Autodesk Inventor part; units mm, degrees
ref_plane "YZ Plane" through (0, 0, 0) normal (1, 0, 0) x (0, 1, 0)
ref_plane "XZ Plane" through (0, 0, 0) normal (0, 1, 0) x (-1, 0, 0)
ref_plane "XY Plane" through (0, 0, 0) normal (0, 0, 1) x (1, 0, 0)
sketch "Sketch1" plane through (0, 0, 0) normal (0, 0, 1) x (1, 0, 0)
  circle A0 centre (12.7, -88.9) radius 2.1844
  circle A1 centre (-149.225, -88.9) radius 2.1844
  circle A2 centre (12.7, -25.4) radius 2.1844
  circle A3 centre (-149.225, -25.4) radius 2.1844
  circle A4 centre (-149.225, -63.5) radius 2.1844
  circle A5 centre (12.7, -63.5) radius 2.1844
  line L0 (12.7, -19.05) -> (-149.225, -19.05)
  line L1 (-155.575, -25.4) -> (-155.575, -98.425)
  line L2 (-152.4, -101.6) -> (-140.7239, -101.6)
  line L3 (-138.1125, -100.2308) -> (-116.4997, -68.9766)
  line L4 (-106.054, -63.5) -> (-30.471, -63.5)
  line L5 (-20.0253, -68.9766) -> (1.5875, -100.2308)
  line L6 (4.1989, -101.6) -> (15.875, -101.6)
  line L7 (19.05, -98.425) -> (19.05, -25.4)
  arc A6 (19.05, -25.4) -> (12.7, -19.05) centre (12.7, -25.4) ccw
  arc A7 (-149.225, -19.05) -> (-155.575, -25.4) centre (-149.225, -25.4) ccw
  arc A8 (15.875, -101.6) -> (19.05, -98.425) centre (15.875, -98.425) ccw
  arc A9 (1.5875, -100.2308) -> (4.1989, -101.6) centre (4.1989, -98.425) ccw
  arc A10 (-140.7239, -101.6) -> (-138.1125, -100.2308) centre (-140.7239, -98.425) ccw
  arc A11 (-155.575, -98.425) -> (-152.4, -101.6) centre (-152.4, -98.425) ccw
  line L8 (-68.2625, -19.05) -> (-68.2625, -63.5) construction
  arc A12 (-20.0253, -68.9766) -> (-30.471, -63.5) centre (-30.471, -76.2) ccw
  arc A13 (-106.054, -63.5) -> (-116.4997, -68.9766) centre (-106.054, -76.2) ccw
  line L9 (-119.0625, -19.05) -> (-119.0625, 0)
  line L10 (-119.0625, 0) -> (-17.4625, 0)
  line L11 (-17.4625, 0) -> (-17.4625, -19.05)
  point P0 (0, 0)
  point P1 (-112.7125, -63.5)
  point P2 (-23.8125, -63.5)
  dimension "d0" = 6.35
  dimension "d2" = 3.175
  dimension "d3" = 12.7
  dimension "d4" = 88.9
  dimension "d5" = 44.45
  dimension "d6" = 25.4
  dimension "d7" = 12.7
  dimension "d23" = 101.6
  dimension "d24" = 19.05
extrude "Extrusion1" add sketch "Sketch1" along normal blind 6.35
fillet "Fillet2" radius 3.175 4 edges at (-119.0625, 0, 3.175) (-119.0625, -19.05, 3.175) (-17.4625, 0, 3.175) (-17.4625, -19.05, 3.175)
sketch "Sketch3" plane through (0, 0, 6.35) normal (0, 0, 1) x (1, 0, 0)
  circle A0 centre (12.7, -25.4) radius 2.1844
  circle A1 centre (12.7, -25.4) radius 4.7625
  circle A2 centre (12.7, -63.5) radius 2.1844
  circle A3 centre (12.7, -63.5) radius 4.7625
  circle A4 centre (-149.225, -25.4) radius 2.1844
  circle A5 centre (-149.225, -25.4) radius 4.7625
  circle A6 centre (-149.225, -63.5) radius 2.1844
  circle A7 centre (-149.225, -63.5) radius 4.7625
  point P0 (0, 0)
  dimension "d26" = 9.525
  dimension "d27" = 9.525
  dimension "d28" = 9.525
  dimension "d29" = 9.525
extrude "Extrusion3" cut sketch "Sketch3" against normal blind 3.175 contours A0 | A1 | A2 | A3 | A4 | A5 | A6 | A7
properties part number "backalignermidgoal" material "Acetal Resin, Black"
For this review, take the finished solid that the model builds, in its own axes (mm). A direction names the side the tool comes from. Round coordinates to 2 decimals unless told otherwise and drop trailing zeros. Write each loop counter-clockwise with the first axis right and the second up, starting at its lowest first coordinate (ties: lowest second). Pieces come first, ordered by that corner, then holes. Notation, with made-up numbers: M -6,33.5 L 19,33.5 A31 ccw 19,57.5 Z; hole C 25.5,2.5 d1. An arc over 180 degrees is marked long. One line per item, written item: value. Start each with the question number.
(1) We need section B-B (z = 4.5). Count the separate pieces of the cut face and the enclosed holes in it, and give its area (3 significant figures).
(2) We need section A-A (y = -79). Give the boundary of the cut face in (x, z) (3 decimals).
(3) The part is to be moulded in two halves that separate along X. For faces 1 (the cylindrical face through (-152.735, -60.281, 4.785)), 2 (the flat face through (-69, -39, 6.35)), 3 (the flat face through (-119.062, -10, 3)), say which applies: released by +X, released by -X, zero draft, split by the parting line, or undercut.
(4) We need section C-C (x = -26). Give the boundary of the cut face in (y, z).
(5) We need section D-D (x = -65). Give the boundary of the cut face in (y, z).
(6) Machinability: for faces 4 (the flat face through (-1, -19.05, 3)), 5 (the flat face through (-136, -19.05, 3)), 6 (the flat face through (-150.35, -27.45, 3.175)), which of the approach directions +Z, -Z, +X, -X, +Y, -Y give a long, thin tool a straight path to every point of the face, cutting with its end or side? Answer none if there is none.
(7) Wall thickness on line 1 (Y direction, x = 12.7, z = 5.2); line 2 (Y direction, x = 12.7, z = 2.25); line 3 (X direction, y = -26.5, z = 5) (3 decimals): over which ranges is each line inside the solid? List them lowest first.
(8) Insertion check: pin 1 (3 mm diameter, centred on y = -8.5, z = 4.5, fed in from -X); pin 2 (5 mm diameter, centred on x = -149.225, y = -63.5, fed in from +Z) (3 decimals); pin 3 (1.5 mm diameter, centred on y = -20.5, z = 3, fed in from -X); pin 4 (3.5 mm diameter, centred on x = 12.7, y = -25.4, fed in from +Z). Each pin has a flat end and moves straight along its axis. Give the tip position at first contact, or say it passes through.
Result:
1. separate pieces: 1
1. enclosed holes: 6
1. area: 11,600 mm²
2. outline: M -155.575,0 L -123.431,0 L -123.431,6.35 L -155.575,6.35 Z; M -13.094,0 L 19.05,0 L 19.05,6.35 L -13.094,6.35 Z
3. face 1: undercut
3. face 2: zero draft
3. face 3: released by -X
4. outline: M -64.31,0 L 0,0 L 0,6.35 L -64.31,6.35 Z
5. outline: M -63.5,0 L 0,0 L 0,6.35 L -63.5,6.35 Z
6. face 4: +Z, -Z, +X, +Y
6. face 5: +Z, -Z, -X, +Y
6. face 6: +Z
7. line 1: -101.6 to -91.08, -86.72 to -68.26, -58.74 to -30.16, -20.64 to -19.05
7. line 2: -101.6 to -91.08, -86.72 to -65.68, -61.32 to -27.58, -23.22 to -19.05
7. line 3: -155.575 to -153.859, -144.591 to 8.066, 17.334 to 19.05
8. pin 1: x = -119.06
8. pin 2: z = 3.175
8. pin 3: x = -154.03
8. pin 4: through
